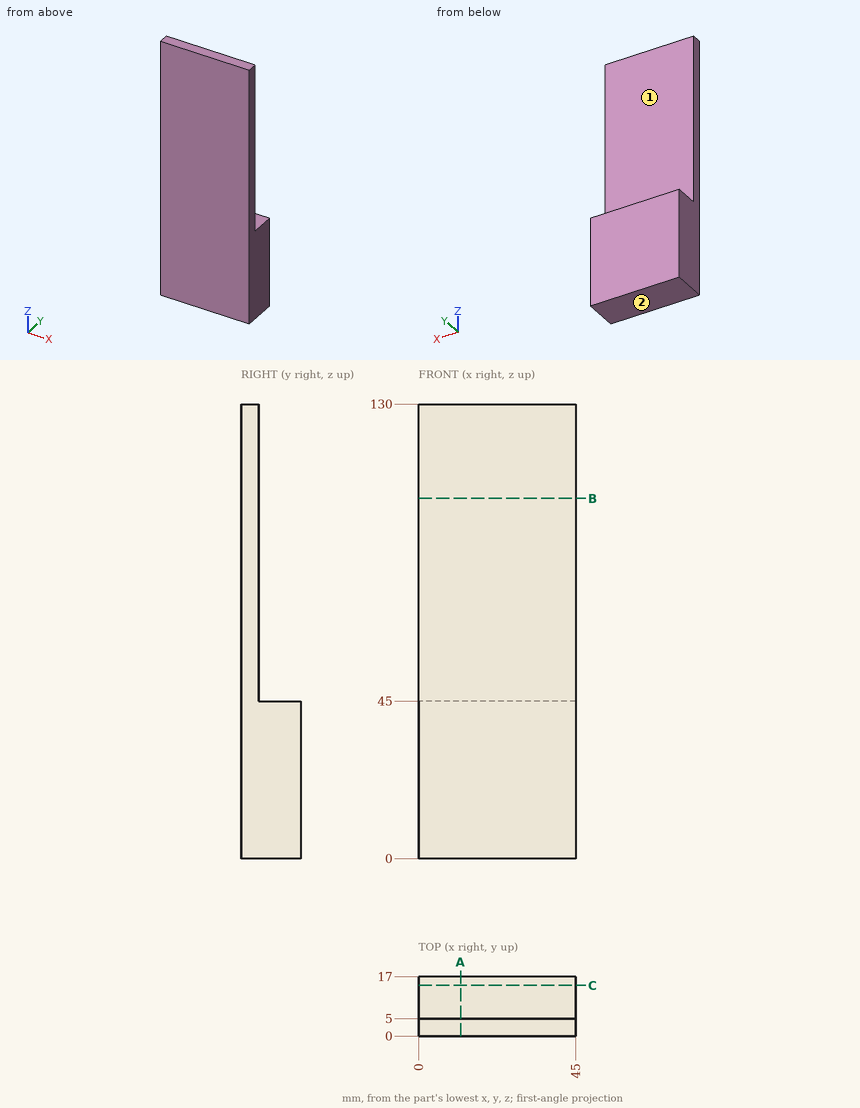
Study the drawing (mm; zero at the part's minimum x, y, z) and answer. A direction names the side the tool comes from. Coordinates: 2 decimals unless noted, no trailing zeros. Loops run counter-clockwise (first coordinate to the right, second up) from the corner with the lowest first, then second, coordinate; pieces in that order, holes last. Notation, with made-up numbers: (-23, 12.25) -> (-19, 12.25) arc R17 ccw to (-19, 36.25) -> close; hole circle Ø1 at (-24, 80). An arc over 180 degrees is marked (long way). Write each question's results on one line, items separated by ' | '. Start each with the question number.
1) For the marked faces 1 and 2, determine the directions among +Z, -Z, +X, -X, +Y, -Y from which every point of the face is accessible in a straight line to the end or side of a thin tool.
2) Find section B-B on z = 103. Determine the outline of the cut face in (x, y).
3) Find section C-C on y = 14.5. Determine the outline of the cut face in (x, z), then the cut area to 4 significant figures.
4) Consider line 1 along Y through (x, z) = (32.5, 90); line 2 along Z through (x, y) = (40, 8.25). Determine where each line is inside the solid, lowest interval first.
5) Find section A-A on x = 12. Determine the outline of the cut face in (y, z), then the cut area to 3 significant figures.
6) Flat-ended cylindrical pins translate along their axes: P1, Ø13.5, axis at x = 21.5, z = 90, coming from the +Y side; P2, Ø6, axis at x = 12.5, y = 12, coming from the +Z side. Find the tip coordinate at first contact, or state that the pin passes through.
Response values:
1) face 1: +Z, +X, -X, +Y | face 2: -Z, +X, -X, +Y, -Y
2) outline: (0, 0) -> (45, 0) -> (45, 5) -> (0, 5) -> close
3) outline: (0, 0) -> (45, 0) -> (45, 45) -> (0, 45) -> close | area: 2,025 mm^2
4) line 1: y = 0 to 5 | line 2: z = 0 to 45
5) outline: (0, 0) -> (17, 0) -> (17, 45) -> (5, 45) -> (5, 130) -> (0, 130) -> close | area: 1,190 mm^2
6) P1: stops at y = 5 | P2: stops at z = 45
